Geometry check sheet. Reference: the model listing, model coordinates, mm. A direction names the side the tool comes from. Round coordinates to 2 decimals unless told otherwise and drop trailing zeros. Write each loop counter-clockwise with the first axis right and the second up, starting at its lowest first coordinate (ties: lowest second). Pieces come first, ordered by that corner, then holes. Notation, with made-up numbers: (36.25, -24.75) - (87.25, -24.75) arc R24 cw to (87.25, -2.75) - close; hole circle Ø3 at (78.25, -38). An arc over 180 degrees is marked (long way). Return JSON: item names as keys, results as strings. Group by question number.
from build123d import *

# Parameters (mm, degrees)
BOSS_EXTRUDE1_DEPTH = 6
SKETCH3_R           = 5
CUT_EXTRUDE1_DEPTH  = 262.076617107
SKETCH4_R           = 5
CUT_EXTRUDE2_DEPTH  = 262.076617107
CUT_EXTRUDE5_DEPTH  = 262.076617107
FILLET5_R           = 5
FILLET6_R           = 5
SKETCH9_W           = 180
SKETCH9_H           = 10
BOSS_EXTRUDE2_DEPTH = 6
CUT_EXTRUDE6_DEPTH  = 262.076617107
FILLET7_R           = 10
SKETCH11_R          = 5
BOSS_EXTRUDE3_DEPTH = 6


with BuildPart() as part:
    # Sketch1 → Boss-Extrude1 (new body)
    with BuildSketch(Plane.XY):
        with BuildLine():
            Line((-250, -55), (-250, 3.178280867))
            Line((-250, 3.178280867), (-250, 55))
            ThreePointArc((-250, 55), (-244.142135624, 69.142135624), (-230, 75))
            Line((-230, 75), (-220, 75))
            Line((-220, 75), (-164.330865428, 75))
            Line((-164.330865428, 75), (-60, 75))
            ThreePointArc((-60, 75), (-52.928932188, 72.071067812), (-50, 65))
            Line((-50, 65), (-50, 20))
            ThreePointArc((-50, 20), (-48.100925873, 14.1369803), (-43.125, 10.500822404))
            ThreePointArc((-43.125, 10.500822404), (-39.437786703, 8.32242004), (-37, 4.801315846))
            ThreePointArc((-37, 4.801315846), (-22.271648276, -13.226099426), (0, -20))
            Line((0, -20), (0, -40))
            Line((0, -40), (0, -65))
            Line((0, -65), (0, -75))
            Line((0, -75), (-230, -75))
            ThreePointArc((-230, -75), (-244.142135624, -69.142135624), (-250, -55))
        make_face()
    boss_extrude1 = extrude(amount=BOSS_EXTRUDE1_DEPTH)

    # Mirror1: Boss-Extrude1 across plane
    add(boss_extrude1.mirror(Plane(origin=(0, -20, 6), x_dir=(0, 0, 1), z_dir=(-1, 0, 0))))

    # Sketch3 → Cut-Extrude1 (cut, through all)
    with BuildSketch(Plane.XY.offset(6)):
        with Locations((110, 55)):
            Circle(SKETCH3_R)
        with Locations((200, 55)):
            Circle(SKETCH3_R)
        with Locations((-110, 55)):
            Circle(SKETCH3_R)
        with Locations((-200, 55)):
            Circle(SKETCH3_R)
    extrude(amount=-CUT_EXTRUDE1_DEPTH, mode=Mode.SUBTRACT)

    # Sketch4 → Cut-Extrude2 (cut, through all)
    with BuildSketch(Plane.XY.offset(6)):
        with BuildLine():
            Line((-70, -55), (-70, 25))
            ThreePointArc((-70, 25), (-72.928932188, 32.071067812), (-80, 35))
            Line((-80, 35), (-110, 35))
            ThreePointArc((-110, 35), (-113.535533906, 33.535533906), (-115, 30))
            Line((-115, 30), (-115, 25))
            ThreePointArc((-115, 25), (-115.614239502, 21.549275456), (-117.381499976, 18.522465177))
            ThreePointArc((-117.381499976, 18.522465177), (-117.5115076, 18.372596167), (-117.644462896, 18.225335882))
            ThreePointArc((-117.644462896, 18.225335882), (-122.017250069, 15.45520022), (-127.189262676, 15.242585951))
            ThreePointArc((-127.189262676, 15.242585951), (-127.232362089, 15.252356208), (-127.275417902, 15.262316838))
            ThreePointArc((-127.275417902, 15.262316838), (-131.839411289, 17.704627959), (-134.570789944, 22.101728126))
            ThreePointArc((-134.570789944, 22.101728126), (-134.892115533, 23.535059632), (-135, 25))
            Line((-135, 25), (-135, 30))
            ThreePointArc((-135, 30), (-136.464466094, 33.535533906), (-140, 35))
            Line((-140, 35), (-215, 35))
            ThreePointArc((-215, 35), (-218.535533906, 33.535533906), (-220, 30))
            Line((-220, 30), (-220, 25))
            ThreePointArc((-220, 25), (-220.586588267, 21.625436392), (-222.277535909, 18.646768667))
            ThreePointArc((-222.277535909, 18.646768667), (-226.488765584, 15.636708224), (-231.640827685, 15.135534251))
            ThreePointArc((-231.640827685, 15.135534251), (-237.629163678, 18.535028107), (-240, 25))
            Line((-240, 25), (-240, -55))
            ThreePointArc((-240, -55), (-237.071067812, -62.071067812), (-230, -65))
            Line((-230, -65), (-210, -65))
            Line((-210, -65), (-190, -65))
            Line((-190, -65), (-110, -65))
            Line((-110, -65), (-90, -65))
            Line((-90, -65), (-80, -65))
            ThreePointArc((-80, -65), (-72.928932188, -62.071067812), (-70, -55))
        make_face()
        with Locations((-230, 25)):
            Circle(SKETCH4_R)
        with Locations((-125, 25)):
            Circle(SKETCH4_R)
    cut_extrude2 = extrude(amount=-CUT_EXTRUDE2_DEPTH, mode=Mode.SUBTRACT)

    # Sketch8 → Cut-Extrude5 (cut, through all)
    with BuildSketch(Plane.XY.offset(6)):
        with BuildLine():
            Line((-60, 0), (-60, -65))
            Line((-60, -65), (60, -65))
            Line((60, -65), (60, 0))
            ThreePointArc((60, 0), (57.236067977, 4.472135955), (52, 4))
            ThreePointArc((52, 4), (49.247332505, 2.266223145), (46.25, 1.001644808))
            ThreePointArc((46.25, 1.001644808), (0, -30), (-46.25, 1.001644808))
            ThreePointArc((-46.25, 1.001644808), (-49.247332505, 2.266223145), (-52, 4))
            ThreePointArc((-52, 4), (-57.236067977, 4.472135955), (-60, 0))
        make_face()
    extrude(amount=-CUT_EXTRUDE5_DEPTH, mode=Mode.SUBTRACT)

    # Fillet5
    fillet5_edges = [part.edges().sort_by_distance(p)[0] for p in [
        (-60, -65, 3),
    ]]
    fillet(fillet5_edges, radius=FILLET5_R)

    # Fillet6
    fillet6_edges = [part.edges().sort_by_distance(p)[0] for p in [
        (60, -65, 3),
    ]]
    fillet(fillet6_edges, radius=FILLET6_R)

    # Mirror2: Cut-Extrude2 across plane
    add(cut_extrude2.mirror(Plane(origin=(0, 0, 0), x_dir=(0, 0, 1), z_dir=(1, 0, 0))), mode=Mode.SUBTRACT)

    # Sketch9 → Boss-Extrude2 (add)
    with BuildSketch(Plane.XY.offset(6)):
        with Locations((-160, 0)):
            Rectangle(SKETCH9_W, SKETCH9_H)
        with Locations((160, 0)):
            Rectangle(SKETCH9_W, SKETCH9_H)
    extrude(amount=-BOSS_EXTRUDE2_DEPTH)

    # Sketch10 → Cut-Extrude6 (cut, through all)
    with BuildSketch(Plane.XY.offset(6)):
        with BuildLine():
            Line((-240, -5), (-250, -5))
            Line((-250, -5), (-250, -80.075651127))
            Line((-250, -80.075651127), (258.523461634, -80.075651127))
            Line((258.523461634, -80.075651127), (258.523461634, -5))
            Line((258.523461634, -5), (43.301270189, -5))
            ThreePointArc((43.301270189, -5), (0, -30), (-43.301270189, -5))
            Line((-43.301270189, -5), (-240, -5))
        make_face()
    extrude(amount=-CUT_EXTRUDE6_DEPTH, mode=Mode.SUBTRACT)

    # Fillet7
    fillet7_edges = [part.edges().sort_by_distance(p)[0] for p in [
        (-60, -5, 3),
        (250, -5, 3),
        (60, -5, 3),
        (-250, -5, 3),
    ]]
    fillet(fillet7_edges, radius=FILLET7_R)

    # Sketch11 → Boss-Extrude3 (add)
    with BuildSketch(Plane.XY.offset(6)):
        with BuildLine():
            ThreePointArc((-195, 30), (-196.464466094, 33.535533906), (-200, 35))
            Line((-200, 35), (-200, 37.801896892))
            Line((-200, 37.801896892), (-80, 37.801896892))
            Line((-80, 37.801896892), (-80, 35))
            ThreePointArc((-80, 35), (-83.535533906, 33.535533906), (-85, 30))
            Line((-85, 30), (-85, 25))
            ThreePointArc((-85, 25), (-95, 15), (-105, 25))
            Line((-105, 25), (-105, 30))
            ThreePointArc((-105, 30), (-106.464466094, 33.535533906), (-110, 35))
            ThreePointArc((-110, 35), (-113.535533906, 33.535533906), (-115, 30))
            Line((-115, 30), (-115, 25))
            ThreePointArc((-115, 25), (-125, 15), (-135, 25))
            Line((-135, 25), (-135, 30))
            ThreePointArc((-135, 30), (-136.464466094, 33.535533906), (-140, 35))
            ThreePointArc((-140, 35), (-143.535533906, 33.535533906), (-145, 30))
            Line((-145, 30), (-145, 25))
            ThreePointArc((-145, 25), (-155, 15), (-165, 25))
            Line((-165, 25), (-165, 30))
            ThreePointArc((-165, 30), (-166.464466094, 33.535533906), (-170, 35))
            ThreePointArc((-170, 35), (-173.535533906, 33.535533906), (-175, 30))
            Line((-175, 30), (-175, 25))
            ThreePointArc((-175, 25), (-185, 15), (-195, 25))
            Line((-195, 25), (-195, 30))
        make_face()
        with Locations((-185, 25)):
            Circle(SKETCH11_R, mode=Mode.SUBTRACT)
        with Locations((-155, 25)):
            Circle(SKETCH11_R, mode=Mode.SUBTRACT)
        with Locations((-95, 25)):
            Circle(SKETCH11_R, mode=Mode.SUBTRACT)
        with Locations((-125, 25)):
            Circle(SKETCH11_R, mode=Mode.SUBTRACT)
    boss_extrude3 = extrude(amount=-BOSS_EXTRUDE3_DEPTH)

    # Mirror3: Boss-Extrude3 across plane
    add(boss_extrude3.mirror(Plane(origin=(0, 0, 0), x_dir=(0, 0, 1), z_dir=(1, 0, 0))))


solid = part.part
1. Tool access check on faces 4 (the face through (-53.01, 72.15, 2.96)), 5 (the face through (-155, 15, 3)), 6 (the face through (52, 35, 6)). Record the directions out of +Z, -Z, +X, -X, +Y, -Y that give a thin tool (end or side, any length) a straight path to the whole face; none if there is none.
2. Section check B-B (z = 3.75). State how many separate pieces and enclosed holes the cut face has, and give its area (3 significant figures).
3. Mould release check, pull along X, two halves, no side actions. Record for faces 1 (the face through (244.297, 68.986, 2.958)), 2 (the face through (-244.297, 68.986, 2.958)), 3 (the face through (203, 59, 3)): pulls with the +X half, pulls with the -X half, needs draft (parallel to the pull), parting line crosses it, or undercut.
4. Depth check by flat-ended pin: pin 1 Ø6 at (x, y) = (-185, 25) entering from +Z; pin 2 Ø1 at (x, z) = (9, 3.5) entering from +Y. Enter the tip coordinate at first touch or a pass-through.
5. Section check A-A (x = -95). Enter the section's corners in (y, z).
6. Section check C-C (x = -185.5). Enter the section's corners in (y, z).
7. Section check D-D (x = 24). Enter the section's corners in (y, z).
8. Material ranges on line 1 along X through (y, z) = (54.5, 5.5); line 2 along Y through (x, z) = (-110, 1.55); line 3 along Y through (x, z) = (206.5, 3.5), recorded low to high.
Result sheet:
{
 "1": {"face 4": "+Z, -Z, +Y", "face 5": "+Z, -Z", "face 6": "+Z, +X, -X, +Y, -Y"},
 "2": {"separate pieces": "1", "enclosed holes": "16", "area": "25,200 mm²"},
 "3": {"face 1": "pulls with the +X half", "face 2": "pulls with the -X half", "face 3": "undercut"},
 "4": {"pin 1": "passes through", "pin 2": "stops at y = -18.86"},
 "5": {"outline": "(-5, 0) - (5, 0) - (5, 6) - (-5, 6) - close; (15, 0) - (20, 0) - (20, 6) - (15, 6) - close; (30, 0) - (75, 0) - (75, 6) - (30, 6) - close"},
 "6": {"outline": "(-5, 0) - (5, 0) - (5, 6) - (-5, 6) - close; (15.01, 0) - (20.03, 0) - (20.03, 6) - (15.01, 6) - close; (29.97, 0) - (75, 0) - (75, 6) - (29.97, 6) - close"},
 "7": {"outline": "(-23.86, 0) - (-12, 0) - (-12, 6) - (-23.86, 6) - close"},
 "8": {"line 1": "x = -250 to -204.97, -195.03 to -114.97, -105.03 to -50, 50 to 105.03, 114.97 to 195.03, 204.97 to 250", "line 2": "y = -5 to 5, 35 to 50, 60 to 75", "line 3": "y = -5 to 5, 35 to 75"}
}
